For this review, take the finished solid that the model builds, in its own axes (mm). Give positions to 0.01 mm unless a question says otherwise; leave off trailing zeros. Order: outer loops, then holes, each group sorted by start corner. A loop starts at its lowest first (then second) coordinate and runs counter-clockwise, first axis right, second up. Notation, with made-up numbers: (71.5, -31.5) - (107.5, -31.5) arc R22 cw to (107.5, -12.5) - close; hole circle Ø6 at (80.25, -35.75). An arc over 180 degrees is marked (long way). Use a Markdown table: item, result. Add a question column.
1) Wall thickness on L1, parallel to X at y = -17.5, z = 0.6; L2, parallel to X at y = -22, z = 1.1; L3, parallel to Y at x = -23.5, z = 0.45: over which ranges is each line inside the solid? List them lowest first.
2) We need section A-A on x = -7.5. Write out the cut boundary in (y, z), then the cut area to 3 significant figures.
3) We need section B-B on z = 1.3. Give the number of separate pieces and of enclosed holes in the cut face, then the cut area to 3 significant figures.
4) We need section C-C on y = -8. Write out the cut boundary in (x, z), then the cut area to 3 significant figures.
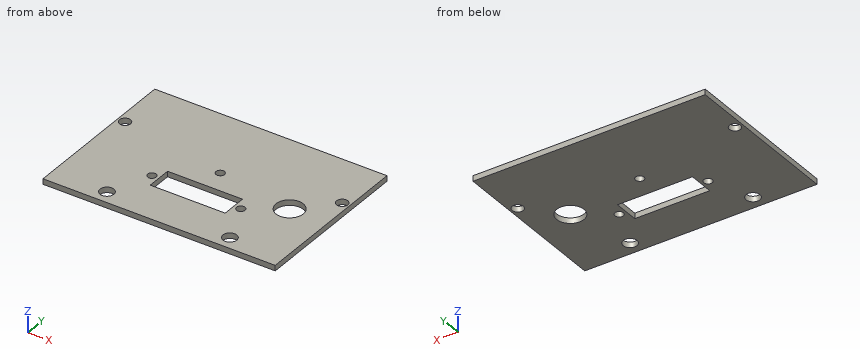
```python
from build123d import *

# Parameters (mm, degrees)
SKETCH1_W           = 85
SKETCH1_H           = 60
BOSS_EXTRUDE1_DEPTH = 2
CUT_EXTRUDE1_REACH  = 4
SKETCH2_R           = 2.55
CUT_EXTRUDE2_REACH  = 4
SKETCH3_R           = 5
SKETCH3_R_2         = 1.55
SKETCH3_W           = 27.44
SKETCH3_H           = 9.3
CUT_EXTRUDE3_REACH  = 4
SKETCH4_R           = 2.05


with BuildPart() as part:
    # Sketch1 → Boss-Extrude1 (new body)
    with BuildSketch(Plane.XY):
        with Locations((-15.192849494, -7.500433728)):
            Rectangle(SKETCH1_W, SKETCH1_H)
    extrude(amount=BOSS_EXTRUDE1_DEPTH)

    # Sketch2 → Cut-Extrude1 (cut, up to next)
    with BuildSketch(Plane(origin=(0, 0, 0), x_dir=(-1, 0, 0), z_dir=(0, 0, -1)), mode=Mode.PRIVATE) as cut_extrude1_sk1:
        with Locations((-7.307150506, -32.500433728)):
            Circle(SKETCH2_R)
    cut_extrude1_tool1 = extrude(cut_extrude1_sk1.sketch, amount=-CUT_EXTRUDE1_REACH, mode=Mode.PRIVATE) & part.part
    add(cut_extrude1_tool1.solids().sort_by_distance((7.307151, -32.500434, 0))[0], mode=Mode.SUBTRACT)
    # Sketch2 → Cut-Extrude1 (cut, up to next)
    with BuildSketch(Plane(origin=(0, 0, 0), x_dir=(-1, 0, 0), z_dir=(0, 0, -1)), mode=Mode.PRIVATE) as cut_extrude1_sk2:
        with Locations((37.692849494, -32.500433728)):
            Circle(SKETCH2_R)
    cut_extrude1_tool2 = extrude(cut_extrude1_sk2.sketch, amount=-CUT_EXTRUDE1_REACH, mode=Mode.PRIVATE) & part.part
    add(cut_extrude1_tool2.solids().sort_by_distance((-37.692849, -32.500434, 0))[0], mode=Mode.SUBTRACT)

    # Sketch3 → Cut-Extrude2 (cut, up to next)
    with BuildSketch(Plane(origin=(0, 0, 0), x_dir=(-1, 0, 0), z_dir=(0, 0, -1)), mode=Mode.PRIVATE) as cut_extrude2_sk1:
        with Locations((-13.307150506, -9.240433728)):
            Circle(SKETCH3_R)
    cut_extrude2_tool1 = extrude(cut_extrude2_sk1.sketch, amount=-CUT_EXTRUDE2_REACH, mode=Mode.PRIVATE) & part.part
    add(cut_extrude2_tool1.solids().sort_by_distance((13.307151, -9.240434, 0))[0], mode=Mode.SUBTRACT)
    # Sketch3 → Cut-Extrude2 (cut, up to next)
    with BuildSketch(Plane(origin=(0, 0, 0), x_dir=(-1, 0, 0), z_dir=(0, 0, -1)), mode=Mode.PRIVATE) as cut_extrude2_sk2:
        with Locations((15.192849494, -4.670433728)):
            Circle(SKETCH3_R_2)
    cut_extrude2_tool2 = extrude(cut_extrude2_sk2.sketch, amount=-CUT_EXTRUDE2_REACH, mode=Mode.PRIVATE) & part.part
    add(cut_extrude2_tool2.solids().sort_by_distance((-15.192849, -4.670434, 0))[0], mode=Mode.SUBTRACT)
    # Sketch3 → Cut-Extrude2 (cut, up to next)
    with BuildSketch(Plane(origin=(0, 0, 0), x_dir=(-1, 0, 0), z_dir=(0, 0, -1)), mode=Mode.PRIVATE) as cut_extrude2_sk3:
        with Locations((-1.067150506, -17.500433728)):
            Circle(SKETCH3_R_2)
    cut_extrude2_tool3 = extrude(cut_extrude2_sk3.sketch, amount=-CUT_EXTRUDE2_REACH, mode=Mode.PRIVATE) & part.part
    add(cut_extrude2_tool3.solids().sort_by_distance((1.067151, -17.500434, 0))[0], mode=Mode.SUBTRACT)
    # Sketch3 → Cut-Extrude2 (cut, up to next)
    with BuildSketch(Plane(origin=(0, 0, 0), x_dir=(-1, 0, 0), z_dir=(0, 0, -1)), mode=Mode.PRIVATE) as cut_extrude2_sk4:
        with Locations((31.452849494, -17.500433728)):
            Circle(SKETCH3_R_2)
    cut_extrude2_tool4 = extrude(cut_extrude2_sk4.sketch, amount=-CUT_EXTRUDE2_REACH, mode=Mode.PRIVATE) & part.part
    add(cut_extrude2_tool4.solids().sort_by_distance((-31.452849, -17.500434, 0))[0], mode=Mode.SUBTRACT)
    # Sketch3 → Cut-Extrude2 (cut, up to next)
    with BuildSketch(Plane(origin=(0, 0, 0), x_dir=(-1, 0, 0), z_dir=(0, 0, -1)), mode=Mode.PRIVATE) as cut_extrude2_sk5:
        with Locations((15.192849494, -17.500433728)):
            Rectangle(SKETCH3_W, SKETCH3_H)
    cut_extrude2_tool5 = extrude(cut_extrude2_sk5.sketch, amount=-CUT_EXTRUDE2_REACH, mode=Mode.PRIVATE) & part.part
    add(cut_extrude2_tool5.solids().sort_by_distance((-15.192849, -17.500434, 0))[0], mode=Mode.SUBTRACT)

    # Sketch4 → Cut-Extrude3 (cut, up to next)
    with BuildSketch(Plane.XY.offset(2), mode=Mode.PRIVATE) as cut_extrude3_sk1:
        with Locations((-54.942849494, 2.499566272)):
            Circle(SKETCH4_R)
    cut_extrude3_tool1 = extrude(cut_extrude3_sk1.sketch, amount=-CUT_EXTRUDE3_REACH, mode=Mode.PRIVATE) & part.part
    add(cut_extrude3_tool1.solids().sort_by_distance((-54.942849, 2.499566, 2))[0], mode=Mode.SUBTRACT)
    # Sketch4 → Cut-Extrude3 (cut, up to next)
    with BuildSketch(Plane.XY.offset(2), mode=Mode.PRIVATE) as cut_extrude3_sk2:
        with Locations((24.557150506, 2.499566272)):
            Circle(SKETCH4_R)
    cut_extrude3_tool2 = extrude(cut_extrude3_sk2.sketch, amount=-CUT_EXTRUDE3_REACH, mode=Mode.PRIVATE) & part.part
    add(cut_extrude3_tool2.solids().sort_by_distance((24.557151, 2.499566, 2))[0], mode=Mode.SUBTRACT)


solid = part.part
```
Checked values:
| question | item | result |
|---|---|---|
| 1 | L1 | -57.69 to -33, -29.9 to -28.91, -1.47 to -0.48, 2.62 to 27.31 |
| 1 | L2 | -57.69 to -28.91, -1.47 to 27.31 |
| 1 | L3 | -37.5 to -22.15, -12.85 to 22.5 |
| 2 | outline | (-37.5, 0) - (-22.15, 0) - (-22.15, 2) - (-37.5, 2) - close; (-12.85, 0) - (22.5, 0) - (22.5, 2) - (-12.85, 2) - close |
| 2 | area | 101 mm² |
| 3 | separate pieces | 1 |
| 3 | enclosed holes | 9 |
| 3 | area | 4,680 mm² |
| 4 | outline | (-57.69, 0) - (8.46, 0) - (8.46, 2) - (-57.69, 2) - close; (18.15, 0) - (27.31, 0) - (27.31, 2) - (18.15, 2) - close |
| 4 | area | 151 mm² |
